Design review of the part built by this model. Coordinates are the model's own, in mm. A direction names the side the tool comes from. Coordinates: 2 decimals unless noted, no trailing zeros. Write each loop counter-clockwise with the first axis right and the second up, starting at its lowest first coordinate (ties: lowest second). Pieces come first, ordered by that corner, then holes.
Q1. Take a section at A-A (x = 36). Give the boundary of the cut face in (y, z).
Q2. Insertion check: pin 1 (4 mm diameter, centred on x = 9.5, y = 3.5, fed in from +Z); pin 2 (10 mm diameter, centred on x = 36.5, z = 25, fed in from -Y); pin 3 (3.5 mm diameter, centred on x = 50.5, z = 2, fed in from -Y); pin 4 (10 mm diameter, centred on y = 30, z = 11, fed in from +X). Each pin has a flat end and moves straight along its axis. Give the tip position at first contact, or say it passes through.
Q3. Take a section at B-B (y = 14). Give the boundary of the cut face in (x, z).
Q4. Mouldability with a two-part tool opening along X and no side actions: class faces 1 (the flat face through (75, 0, 4)), 2 (the flat face through (80, 24, 22)), 3 (the flat face through (60, 45, 41)) as pulls with the +X half, pulls with the -X half, needs draft (parallel to the pull), parting line crosses it, or undercut.
Q5. Machinability: for faces 4 (the flat face through (20, 45, 1)), 5 (the flat face through (66, 3, 4)), 6 (the flat face through (14.584, 45.07, 36.824)), which of the approach directions +Z, -Z, +X, -X, +Y, -Y give a long, thin tool a straight path to every point of the face, cutting with its end or side? Answer none if there is none.
Q6. Take a section at D-D (y = 19.5). Give the boundary of the cut face in (x, z).
Q7. Take a section at C-C (x = 64.5). Give the boundary of the cut face in (y, z), and give its area (3 significant figures).
Q8. For probe 1 along Y at (x, z) = (70, 1.05); probe 2 along X at (y, z) = (25, 2.5); probe 3 along Y at (x, z) = (72.5, 21.5), list the stretches that pass through material, from the lowest coordinate up.
```python
from build123d import *

# Parameters (mm, degrees)
EXTRUDE_2_DEPTH     = 2
SKETCH_3_R          = 1.5
CUT_EXTRUDE_1_DEPTH = 95.361008897
EXTRUDE_3_DEPTH     = 1
DRAFT_4_ANGLE       = 43
SKETCH_6_W          = 6
SKETCH_6_H          = 10
EXTRUDE_4_DEPTH     = 5
SKETCH_7_W          = 6
SKETCH_7_H          = 10
EXTRUDE_5_DEPTH     = 5
CUT_EXTRUDE_2_DEPTH = 107.596038813
CUT_EXTRUDE_4_DEPTH = 107.596038813
CUT_EXTRUDE_5_DEPTH = 107.596038813
CUT_EXTRUDE_6_DEPTH = 107.596038813
SKETCH_15_W         = 30
SKETCH_15_H         = 20
CUT_EXTRUDE_7_DEPTH = 107.596038813
SKETCH_16_W         = 20
SKETCH_16_H         = 20
CUT_EXTRUDE_8_DEPTH = 5
SKETCH_17_W         = 15
SKETCH_17_H         = 25
CUT_EXTRUDE_9_DEPTH = 5


with BuildPart() as part:
    # 草图1 → 凸台-拉伸2 (new body)
    with BuildSketch(Plane.XY):
        Polygon((0, 0), (0, 50), (20, 50), (20, 40), (60, 40), (60, 50), (80, 50), (80, 0), (60, 0), (60, 10), (20, 10), (20, 0), align=None)
    extrude(amount=EXTRUDE_2_DEPTH)

    # 草图3 → 切除-拉伸1 (cut, through all)
    with BuildSketch(Plane.XY.offset(2)):
        with Locations((10, 45)):
            Circle(SKETCH_3_R)
        with Locations((10, 5)):
            Circle(SKETCH_3_R)
        with Locations((70, 45)):
            Circle(SKETCH_3_R)
        with Locations((70, 5)):
            Circle(SKETCH_3_R)
    extrude(amount=-CUT_EXTRUDE_1_DEPTH, mode=Mode.SUBTRACT)

    # 草图5 → 凸台-拉伸3 (add)
    with BuildSketch(Plane.XY.offset(2)):
        with BuildLine():
            Line((0, 50), (6, 50))
            Line((6, 50), (6, 45))
            ThreePointArc((6, 45), (10, 41), (14, 45))
            Line((14, 45), (14, 50))
            Line((14, 50), (20, 50))
            Line((20, 50), (20, 40))
            Line((20, 40), (60, 40))
            Line((60, 40), (60, 50))
            Line((60, 50), (66, 50))
            Line((66, 50), (66, 45))
            ThreePointArc((66, 45), (70, 41), (74, 45))
            Line((74, 45), (74, 50))
            Line((74, 50), (80, 50))
            Line((80, 50), (80, 0))
            Line((80, 0), (74, 0))
            Line((74, 0), (74, 5))
            ThreePointArc((74, 5), (70, 9), (66, 5))
            Line((66, 5), (66, 0))
            Line((66, 0), (60, 0))
            Line((60, 0), (60, 10))
            Line((60, 10), (20, 10))
            Line((20, 10), (20, 0))
            Line((20, 0), (14, 0))
            Line((14, 0), (14, 5))
            ThreePointArc((14, 5), (10, 9), (6, 5))
            Line((6, 5), (6, 0))
            Line((6, 0), (0, 0))
            Line((0, 0), (0, 50))
        make_face()
    extrude(amount=EXTRUDE_3_DEPTH)

    # 拔模4
    draft_4_faces = [part.faces().sort_by_distance(p)[0] for p in [
        (40, 25, 3),
    ]]
    draft(draft_4_faces, Plane(origin=(20, 0, 2), x_dir=(-1, 0, 0), z_dir=(0, -1, 0)), DRAFT_4_ANGLE)

    # 草图6 → 凸台-拉伸4 (add)
    with BuildSketch(Plane(origin=(0, -1.496346075, 1.604634711), x_dir=(1, 0, 0), z_dir=(0, -0.6819983600624997, 0.7313537016191695))):
        with Locations((3, 7.04599508)):
            Rectangle(SKETCH_6_W, SKETCH_6_H)
    extrude(amount=EXTRUDE_4_DEPTH)

    # 草图7 → 凸台-拉伸5 (add)
    with BuildSketch(Plane(origin=(0, -1.496346075, 1.604634711), x_dir=(1, 0, 0), z_dir=(0, -0.6819983600624997, 0.7313537016191695))):
        with Locations((77, 7.04599508)):
            Rectangle(SKETCH_7_W, SKETCH_7_H)
    extrude(amount=EXTRUDE_5_DEPTH)

    # 草图8 → 切除-拉伸2 (cut, through all)
    with BuildSketch(Plane(origin=(80, 0, 0), x_dir=(0, 0, -1), z_dir=(1, 0, 0))):
        Polygon((-3, 0), (-9.836637305, 0), (-6.656768508, -3.4099918), align=None)
    extrude(amount=-CUT_EXTRUDE_2_DEPTH, mode=Mode.SUBTRACT)

    # 草图11 → 切除-拉伸4 (cut, through all)
    with BuildSketch(Plane(origin=(80, 0, 0), x_dir=(0, 0, -1), z_dir=(1, 0, 0))):
        Polygon((-3, 37), (-3, 13), (-11.020713736, 13), (-33.401075804, 37), align=None)
    extrude(amount=-CUT_EXTRUDE_4_DEPTH, mode=Mode.SUBTRACT)

    # 草图12 → 切除-拉伸5 (cut, through all)
    with BuildSketch(Plane(origin=(80, 0, 0), x_dir=(0, 0, -1), z_dir=(1, 0, 0))):
        Polygon((-3, 50), (-41.42178954, 50), (-32.096638679, 40), (-3, 40), align=None)
    extrude(amount=-CUT_EXTRUDE_5_DEPTH, mode=Mode.SUBTRACT)

    # 草图14 → 切除-拉伸6 (cut, through all)
    with BuildSketch(Plane(origin=(80, 0, 0), x_dir=(0, 0, -1), z_dir=(1, 0, 0))):
        Polygon((-11.020713736, 13), (-3, 4.398837557), (-3, 13), align=None)
    extrude(amount=-CUT_EXTRUDE_6_DEPTH, mode=Mode.SUBTRACT)

    # 草图15 → 切除-拉伸7 (cut, through all)
    with BuildSketch(Plane(origin=(0, 0, 0), x_dir=(-1, 0, 0), z_dir=(0, 0, -1))):
        with Locations((-40, 25)):
            Rectangle(SKETCH_15_W, SKETCH_15_H)
    extrude(amount=-CUT_EXTRUDE_7_DEPTH, mode=Mode.SUBTRACT)

    # 草图16 → 切除-拉伸8 (cut)
    with BuildSketch(Plane(origin=(0, 0, 0), x_dir=(-1, 0, 0), z_dir=(0, 0, -1))):
        with Locations((-15, 25)):
            Rectangle(SKETCH_16_W, SKETCH_16_H)
        with Locations((-65, 25)):
            Rectangle(SKETCH_16_W, SKETCH_16_H)
    extrude(amount=-CUT_EXTRUDE_8_DEPTH, mode=Mode.SUBTRACT)

    # 草图17 → 切除-拉伸9 (cut)
    with BuildSketch(Plane(origin=(0, 40, 0), x_dir=(1, 0, 0), z_dir=(0, 1, 0))):
        with Locations((52.5, -17.5)):
            Rectangle(SKETCH_17_W, SKETCH_17_H)
        with Locations((27.5, -17.5)):
            Rectangle(SKETCH_17_W, SKETCH_17_H)
    extrude(amount=-CUT_EXTRUDE_9_DEPTH, mode=Mode.SUBTRACT)


solid = part.part
```
Response:
1. outline: (10, 0) - (15, 0) - (15, 3) - (10, 3) - close; (10, 8.22) - (15, 12.89) - (15, 16.99) - (10, 12.33) - close; (35, 0) - (40, 0) - (40, 40.3) - (35, 35.64) - (35, 31.54) - (37, 33.4) - (37, 3) - (35, 3) - close
2. pin 1: stops at z = 2
2. pin 2: stops at y = 37
2. pin 3: stops at y = 10
2. pin 4: passes through
3. outline: (0, 0) - (80, 0) - (80, 3) - (0, 3) - close; (0, 11.95) - (80, 11.95) - (80, 16.06) - (0, 16.06) - close
4. face 1: needs draft
4. face 2: pulls with the +X half
4. face 3: undercut
5. face 4: +Z, -Z, +Y
5. face 5: +Z, -Y
5. face 6: +X, -X, +Y
6. outline: (0, 0) - (5, 0) - (5, 3) - (0, 3) - close; (0, 17.08) - (25, 17.08) - (25, 21.18) - (0, 21.18) - close; (55, 17.08) - (80, 17.08) - (80, 21.18) - (55, 21.18) - close; (75, 0) - (80, 0) - (80, 3) - (75, 3) - close
7. outline: (0, 0) - (15, 0) - (15, 3) - (4.4, 3) - (37, 33.4) - (37, 3) - (35, 3) - (35, 0) - (50, 0) - (50, 3) - (40, 3) - (40, 32.1) - (50, 41.42) - (50, 49.63) - (0, 3) - close
7. area: 422 mm2
8. probe 1: y = 0 to 3.5, 6.5 to 15, 35 to 43.5, 46.5 to 50
8. probe 2: x = 0 to 5, 75 to 80
8. probe 3: y = 19.84 to 24.24, 37 to 40
